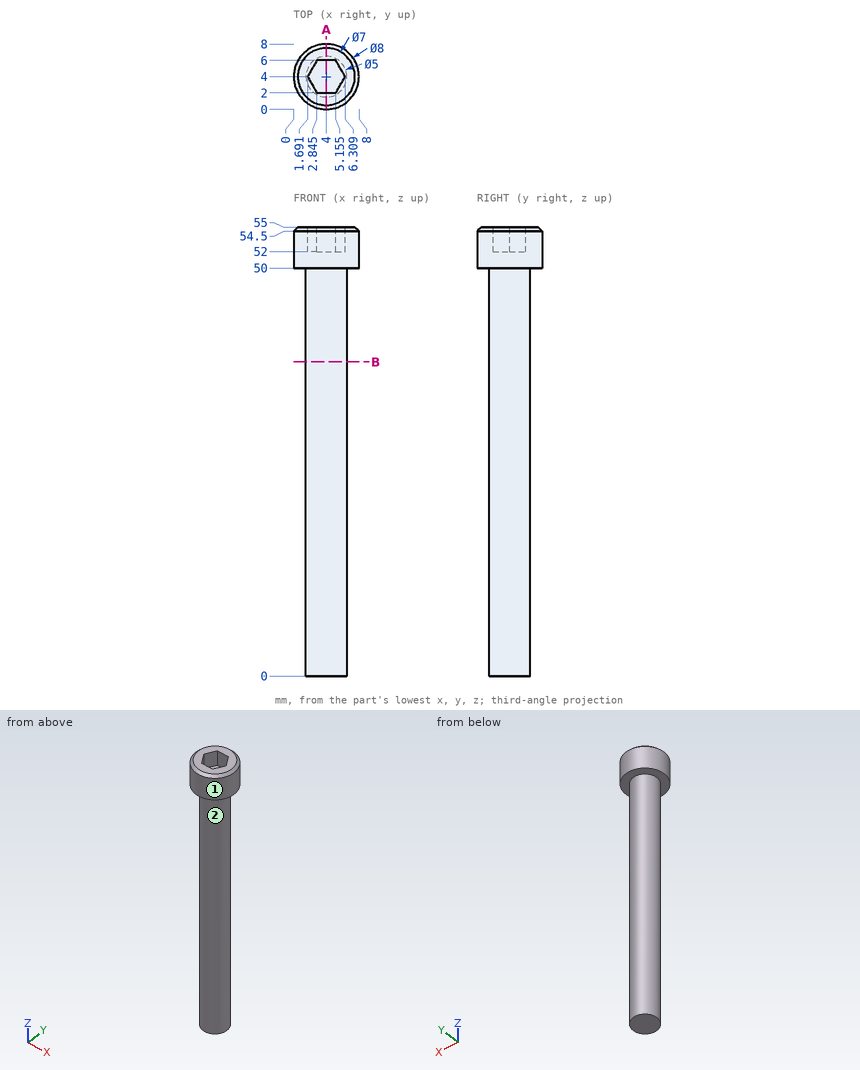
The figure shows three views and two pictorial views of one solid part (mm, origin at its lowest corner). Answer the questions. A direction names the side the tool comes from. Coordinates: 2 decimals unless noted, no trailing zeros. Loops run counter-clockwise (first coordinate to the right, second up) from the corner with the lowest first, then second, coordinate; pieces in that order, holes last. Notation, with made-up numbers: (-1.5, -19.5) -> (25.5, -19.5) arc R22 cw to (25.5, -0.5) -> close; hole circle Ø9 at (-4, 22.5). An arc over 180 degrees is marked (long way). Use one line per item in the form item = value. Start each with the question number.
Item 1: A tool of negligible diameter and unlimited length cuts with its end or side. For the marked faces 1 and 2, from which of +Z, -Z, +X, -X, +Y, -Y can it reach the whole face along a straight path? Write none if from no direction.
Item 2: The part is cut by section B-B on z = 38.5. Determine the outline of the cut face in (x, y), then the cut area to 3 significant figures.
Item 3: The part is cut by section A-A on x = 4. Determine the outline of the cut face in (y, z), then the cut area to 3 significant figures.
Item 4: Consider L1, parallel to Z at x = 3.5, y = 3.25; L2, parallel to Z at x = 6.5, y = 2.25; L3, parallel to Y at x = 2.5, z = 45.5. Determine where each line is inside the solid, lowest interval first. Write a range as [from, to].
Item 5: Flat-ended cylindrical pins translate along their axes: pin 1 Ø2 at (x, y) = (5, 4) entering from +Z; pin 2 Ø1.5 at (x, z) = (7, 33.5) entering from -Y; pin 3 Ø1 at (y, z) = (5, 22) entering from +X. Find the tip coordinate at first contact, or state that the pin passes through.
Answer key:
q1.face_1 = +Z, -Z
q1.face_2 = -Z
q2.outline = circle Ø5 at (4, 4)
q2.area = 19.6 mm2
q3.outline = (0, 50) -> (1.5, 50) -> (1.5, 0) -> (6.5, 0) -> (6.5, 50) -> (8, 50) -> (8, 54.5) -> (7.5, 55) -> (6, 55) -> (6, 52) -> (2, 52) -> (2, 55) -> (0.5, 55) -> (0, 54.5) -> close
q3.area = 278 mm2
q4.L1 = [0, 52]
q4.L2 = [50, 55]
q4.L3 = [2, 6]
q5.pin_1 = 52
q5.pin_2 = 2.91
q5.pin_3 = 6.45
